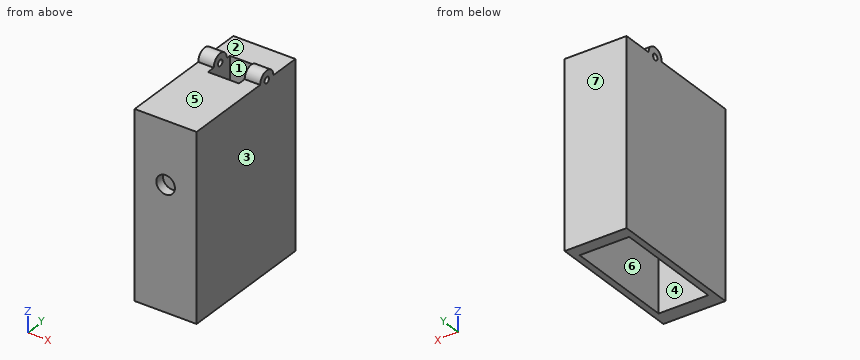
from build123d import *
from build123d.topology import SkipClean

# Parameters (mm, degrees)
BOSS_EXTRUDE2_DEPTH      = 50
BOSS_EXTRUDE2_DEPTH_BACK = 0.0001
SKETCH5_W                = 20
SKETCH5_H                = 59.382936356
SKETCH6_R                = 5
CUT_EXTRUDE1_DEPTH       = 45
SKETCH9_W                = 10
SKETCH9_H                = 10
CUT_EXTRUDE4_DEPTH       = 0.076800532
BOSS_EXTRUDE5_DEPTH      = 5
CUT_EXTRUDE6_DEPTH       = 5
BOSS_EXTRUDE6_START      = -5
BOSS_EXTRUDE6_DEPTH      = 5
SKETCH15_R               = 1
CUT_EXTRUDE7_DEPTH       = 20
SKETCH19_R               = 5
BOSS_EXTRUDE13_DEPTH     = 45
BOSS_EXTRUDE15_DEPTH     = 5
SKETCH22_R               = 1
CUT_EXTRUDE8_DEPTH       = 5
BOSS_EXTRUDE16_START     = -5
BOSS_EXTRUDE16_DEPTH     = 5
SKETCH24_W               = 15.993114704
SKETCH24_H               = 35.984045661
CUT_EXTRUDE9_DEPTH       = 36
SKETCH26_W               = 10
SKETCH26_H               = 10
CUT_EXTRUDE13_DEPTH      = 36
CUT_EXTRUDE14_DEPTH      = 5
SKETCH29_W               = 20.000394844
SKETCH29_H               = 5
CUT_EXTRUDE15_DEPTH      = 1
SKETCH31_R               = 3
CUT_EXTRUDE16_DEPTH      = 3
SKETCH32_W               = 19.994111152
SKETCH32_H               = 5
CUT_EXTRUDE17_DEPTH      = 19
SKETCH33_W               = 19.589439069
SKETCH33_H               = 5
CUT_EXTRUDE18_DEPTH      = 19


with BuildPart() as part:
    # Sketch5 → Boss-Extrude2 (new, two sides: drawn at the far end of the back side and taken through both)
    with BuildSketch(Plane(origin=(0.323578151, 0, -7.846011644), x_dir=(1, 0, 0), z_dir=(0, 1, 0)).offset(-BOSS_EXTRUDE2_DEPTH_BACK)):
        with Locations((-45.061859189, 16.472889188)):
            Rectangle(SKETCH5_W, SKETCH5_H)
    extrude(amount=BOSS_EXTRUDE2_DEPTH + BOSS_EXTRUDE2_DEPTH_BACK)

    # Sketch6 → Cut-Extrude1 (cut)
    with BuildSketch(Plane(origin=(0.323578151, 50, -7.846011644), x_dir=(1, 0, 0), z_dir=(0, 1, 0))):
        with Locations(Location((-45.061859189, 16.574918296, 0), (0, 0, 270))):
            Circle(SKETCH6_R)
    extrude(amount=-CUT_EXTRUDE1_DEPTH, mode=Mode.SUBTRACT)

    # Sketch9 → Cut-Extrude4 (cut)
    with BuildSketch(Plane(origin=(0.323578151, 0, 5.372567346), x_dir=(1, 0, 0), z_dir=(0, 0, 1))):
        with Locations((-45.061859189, 36.348822535)):
            Rectangle(SKETCH9_W, SKETCH9_H)
    extrude(amount=-CUT_EXTRUDE4_DEPTH, mode=Mode.SUBTRACT)

    # Sketch10 → Boss-Extrude5 (add)
    with BuildSketch(Plane(origin=(-34.738281038, 0, -7.846011644), x_dir=(0, 0, -1), z_dir=(1, 0, 0))):
        with BuildLine():
            Line((-13.21857899, 38.972016939), (-13.21857899, 34.972016939))
            ThreePointArc((-13.21857899, 34.972016939), (-15.21857899, 36.972016939), (-13.21857899, 38.972016939))
        make_face()
    extrude(amount=-BOSS_EXTRUDE5_DEPTH)

    # Sketch12 → Cut-Extrude6 (cut)
    with BuildSketch(Plane(origin=(-34.738281038, 0, -7.846011644), x_dir=(0, 0, -1), z_dir=(1, 0, 0))):
        with BuildLine():
            Line((-13.21857899, 37.972016939), (-13.21857899, 35.972016939))
            ThreePointArc((-13.21857899, 35.972016939), (-14.21857899, 36.972016939), (-13.21857899, 37.972016939))
        make_face()
    extrude(amount=-CUT_EXTRUDE6_DEPTH, mode=Mode.SUBTRACT)

    # Sketch14 → Boss-Extrude6 (add)
    with BuildSketch(Plane(origin=(-54.738281038, 0, -7.846011644), x_dir=(0, 0, 1), z_dir=(-1, 0, 0)).offset(BOSS_EXTRUDE6_START)):
        with BuildLine():
            Line((13.21857899, 37.972016939), (13.21857899, 38.972016939))
            ThreePointArc((13.21857899, 38.972016939), (15.21857899, 36.972016939), (13.21857899, 34.972016939))
            Line((13.21857899, 34.972016939), (13.21857899, 35.972016939))
            ThreePointArc((13.21857899, 35.972016939), (14.21857899, 36.972016939), (13.21857899, 37.972016939))
        make_face()
    extrude(amount=BOSS_EXTRUDE6_DEPTH)

    # Sketch15 → Cut-Extrude7 (cut)
    with BuildSketch(Plane(origin=(-34.738281038, 0, -7.846011644), x_dir=(0, 0, -1), z_dir=(1, 0, 0))):
        with Locations((-13.21857899, 36.972016939)):
            Circle(SKETCH15_R)
    extrude(amount=-CUT_EXTRUDE7_DEPTH, mode=Mode.SUBTRACT)

    # Sketch19 → Boss-Extrude13 (add)
    with BuildSketch(Plane(origin=(0.323578151, 50, -7.846011644), x_dir=(1, 0, 0), z_dir=(0, 1, 0))):
        with Locations((-45.061859189, 16.574918296)):
            Circle(SKETCH19_R)
    extrude(amount=-BOSS_EXTRUDE13_DEPTH)

    # Sketch21 → Boss-Extrude15 (add)
    with SkipClean():  # the faces are left unmerged after this step: merging them gives an invalid solid
        with BuildSketch(Plane(origin=(-34.738281038, 0, -7.846011644), x_dir=(0, 0, -1), z_dir=(1, 0, 0))):
            with BuildLine():
                Line((-13.21857899, 39.972016939), (-13.21857899, 37.972016939))
                ThreePointArc((-13.21857899, 37.972016939), (-12.21857899, 36.972016939), (-13.21857899, 35.972016939))
                Line((-13.21857899, 35.972016939), (-13.21857899, 33.972016939))
                ThreePointArc((-13.21857899, 33.972016939), (-16.21857899, 36.972016939), (-13.21857899, 39.972016939))
            make_face()
        extrude(amount=-BOSS_EXTRUDE15_DEPTH)

    # Sketch22 → Cut-Extrude8 (cut)
    with BuildSketch(Plane(origin=(-34.738281038, 0, -7.846011644), x_dir=(0, 0, -1), z_dir=(1, 0, 0))):
        with Locations((-13.21857899, 36.972016939)):
            Circle(SKETCH22_R)
    extrude(amount=-CUT_EXTRUDE8_DEPTH, mode=Mode.SUBTRACT)

    # Sketch23 → Boss-Extrude16 (add)
    with BuildSketch(Plane(origin=(-54.738281038, 0, -7.846011644), x_dir=(0, 0, 1), z_dir=(-1, 0, 0)).offset(BOSS_EXTRUDE16_START)):
        with BuildLine():
            Line((13.21857899, 39.972016939), (13.21857899, 37.972016939))
            ThreePointArc((13.21857899, 37.972016939), (14.21857899, 36.972016939), (13.21857899, 35.972016939))
            Line((13.21857899, 35.972016939), (13.21857899, 33.972016939))
            ThreePointArc((13.21857899, 33.972016939), (16.21857899, 36.972016939), (13.21857899, 39.972016939))
        make_face()
    extrude(amount=BOSS_EXTRUDE16_DEPTH)

    # Sketch24 → Cut-Extrude9 (cut)
    with SkipClean():  # the faces are left unmerged after this step: merging them gives an invalid solid
        with BuildSketch(Plane(origin=(0.323578151, 0, -54.01036901), x_dir=(-1, 0, 0), z_dir=(0, 0, -1))):
            with Locations((45.058416541, 28.00797717)):
                Rectangle(SKETCH24_W, SKETCH24_H)
        extrude(amount=-CUT_EXTRUDE9_DEPTH, mode=Mode.SUBTRACT)

    # Sketch26 → Cut-Extrude13 (cut)
    with SkipClean():  # the faces are left unmerged after this step: merging them gives an invalid solid
        with BuildSketch(Plane(origin=(0.323578151, 0, 5.295766814), x_dir=(1, 0, 0), z_dir=(0, 0, 1))):
            with Locations((-45.061859189, 36.348822535)):
                Rectangle(SKETCH26_W, SKETCH26_H)
        extrude(amount=-CUT_EXTRUDE13_DEPTH, mode=Mode.SUBTRACT)

    # Sketch28 → Cut-Extrude14 (cut)
    with SkipClean():  # the faces are left unmerged after this step: merging them gives an invalid solid
        with BuildSketch(Plane(origin=(0, -0.0001, -2.541953713), x_dir=(-1, 0, 0), z_dir=(0, -1, 0))):
            Polygon((54.738281038, -7.914521059), (34.738281038, -7.914521059), (34.738281038, 31.753302396), (54.738281038, 31.878976227), align=None)
        extrude(amount=-CUT_EXTRUDE14_DEPTH, mode=Mode.SUBTRACT)

    # Sketch29 → Cut-Extrude15 (cut)
    with SkipClean():  # the faces are left unmerged after this step: merging them gives an invalid solid
        with BuildSketch(Plane(origin=(0.1981485, 0, -34.075726363), x_dir=(0.9999802581949765, 0, 0.006283567482586401), z_dir=(-0.006283567482586401, 0, 0.9999802581949766))):
            with Locations((-44.937316682, 2.4999)):
                Rectangle(SKETCH29_W, SKETCH29_H)
        extrude(amount=-CUT_EXTRUDE15_DEPTH, mode=Mode.SUBTRACT)

    # Sketch31 → Cut-Extrude16 (cut)
    with SkipClean():  # the faces are left unmerged after this step: merging them gives an invalid solid
        with BuildSketch(Plane(origin=(0, 4.9999, -2.541953713), x_dir=(-1, 0, 0), z_dir=(0, -1, 0))):
            with Locations(Location((44.738281038, 11.982227584, 0), (0, 0, 90))):
                Circle(SKETCH31_R)
        extrude(amount=-CUT_EXTRUDE16_DEPTH, mode=Mode.SUBTRACT)

    # Sketch32 → Cut-Extrude17 (cut)
    with SkipClean():  # the faces are left unmerged after this step: merging them gives an invalid solid
        with BuildSketch(Plane(origin=(0.22040429, 0, -35.075606257), x_dir=(0.9999802581949765, 0, 0.0062835674825864034), z_dir=(-0.0062835674825864034, 0, 0.9999802581949766))):
            with Locations((-44.956431065, 2.4999)):
                Rectangle(SKETCH32_W, SKETCH32_H)
        extrude(amount=-CUT_EXTRUDE17_DEPTH, mode=Mode.SUBTRACT)

    # Sketch33 → Cut-Extrude18 (cut)
    with SkipClean():  # the faces are left unmerged after this step: merging them gives an invalid solid
        with BuildSketch(Plane.ZY.offset(54.738281038)):
            with Locations((-44.215649476, 2.4999)):
                Rectangle(SKETCH33_W, SKETCH33_H)
        extrude(amount=-CUT_EXTRUDE18_DEPTH, mode=Mode.SUBTRACT)


solid = part.part
Could you check a few things on this model? Use its own coordinates, in mm. Face numbers are marked on the shaded views. A direction names the side the tool comes from. Coordinates: 2 decimals unless noted, no trailing zeros. Write each loop counter-clockwise with the first axis right and the second up, starting at its lowest first coordinate (ties: lowest second). Pieces come first, ordered by that corner, then holes. Notation, with made-up numbers: (54, 3.25) - (113, 3.25) arc R30 cw to (113, 42.25) - close; hole circle Ø10 at (-21, -16.75). An arc over 180 degrees is marked (long way). Write item = value, one per line.
1) Suppose I cut it at C-C on y = 22. Please give me the cut outline in (x, z), plus the area to 3 significant figures.
Result set:
outline = (-54.74, -54.01) - (-52.73, -54.01) - (-52.73, -18.01) - (-36.74, -18.01) - (-36.74, -54.01) - (-34.74, -54.01) - (-34.74, 5.37) - (-54.74, 5.37) - close
area = 612 mm2
2) Suppose I cut it at B-B on x = -47. Please give me the cut outline in (y, z), plus the area to 3 significant figures.
Result set:
outline = (5, -54.01) - (10.02, -54.01) - (10.02, -18.01) - (31.35, -18.01) - (31.35, 5.37) - (5, 5.37) - (5, -12.55) - (8, -12.55) - (8, -16.5) - (5, -16.5) - close; (41.35, -18.01) - (46, -18.01) - (46, -54.01) - (50, -54.01) - (50, 5.37) - (41.35, 5.37) - close
area = 1,130 mm2
3) Please list where these lines run through material, in increasing order: line 1 (Y direction, x = -39.25, z = -38); line 2 (X direction, y = 14.5, z = -49); line 3 (Z direction, x = -39.5, y = 37). Write a range as [from, to].
Result set:
line_1 = [5, 10.02], [46, 50]
line_2 = [-54.74, -52.73], [-36.74, -34.74]
line_3 = [-18.01, 4.37], [6.37, 8.37]
4) For the marked faces 1, 2, 3 and 4, which set-ups out of +Z, -Z, +X, -X, +Y, -Y let a thin tool reach every point of the face, with its end or its side?
Result set:
face_1 = +Z, -Z
face_2 = +Z, +X, -X, +Y
face_3 = +Z, -Z, +X, +Y, -Y
face_4 = -Z
5) Suppose I cut it at D-D on x = -51. Please give me the cut outline in (y, z), plus the area to 3 significant figures.
Result set:
outline = (5, -54.01) - (10.02, -54.01) - (10.02, -18.01) - (46, -18.01) - (46, -54.01) - (50, -54.01) - (50, 5.37) - (39.97, 5.37) arc R3 ccw to (33.97, 5.37) - (5, 5.37) - close; hole circle Ø2 at (36.97, 5.37)
area = 1,390 mm2
6) Suppose I cut it at A-A on z = -30. Please give me the cut outline in (x, y), plus the area to 3 significant figures.
Result set:
outline = (-54.74, 5) - (-34.74, 5) - (-34.74, 50) - (-54.74, 50) - close; hole (-52.73, 10.02) - (-36.74, 10.02) - (-36.74, 46) - (-52.73, 46) - close
area = 325 mm2
7) Will these pins go through, and if not, where does the flat tip stop? pin 1 Ø3 at (x, y) = (-44, 39) entering from +Z; pin 2 Ø10 at (x, y) = (-37.5, 25) entering from +Z; pin 3 Ø4 at (x, y) = (-45, 21.5) entering from -Z.
Result set:
pin_1 = through
pin_2 = 5.37
pin_3 = -18.01
8) We'd pull the mould along Y, two halves only. Please class the marked faces 5, 6 and 7: +Y half, -Y half, draft (parallel to the pull), parting line (faces both ways), or undercut.
Result set:
face_5 = draft
face_6 = undercut
face_7 = +Y half
